from build123d import *

# Parameters (mm, degrees)
SKETCH1_R           = 12
BOSS_EXTRUDE1_DEPTH = 20
CUT_EXTRUDE1_DEPTH  = 13
SKETCH3_R           = 3
CUT_EXTRUDE2_DEPTH  = 13


with BuildPart() as part:
    # Sketch1 → Boss-Extrude1 (new body)
    with BuildSketch(Plane(origin=(0, 0, 0), x_dir=(1, 0, 0), z_dir=(0, 1, 0))):
        with Locations(Location((0, 0, 0), (0, 0, 270))):
            Circle(SKETCH1_R)
    extrude(amount=BOSS_EXTRUDE1_DEPTH)

    # Sketch2 → Cut-Extrude1 (cut)
    with BuildSketch(Plane.XZ):
        with BuildLine():
            Line((3.05, 2.739981752), (3.05, -2.739981752))
            ThreePointArc((3.05, -2.739981752), (-4.1, 0), (3.05, 2.739981752))
        make_face()
    extrude(amount=-CUT_EXTRUDE1_DEPTH, mode=Mode.SUBTRACT)

    # Sketch3 → Cut-Extrude2 (cut)
    with BuildSketch(Plane(origin=(0, 20, 0), x_dir=(1, 0, 0), z_dir=(0, 1, 0))):
        with Locations(Location((0, 0, 0), (0, 0, 270))):
            Circle(SKETCH3_R)
    extrude(amount=-CUT_EXTRUDE2_DEPTH, mode=Mode.SUBTRACT)


solid = part.part
Design review of the part built by this model. Coordinates are the model's own, in mm. A direction names the side the tool comes from. Round coordinates to 2 decimals unless told otherwise and drop trailing zeros. Loops run counter-clockwise (first coordinate to the right, second up) from the corner with the lowest first, then second, coordinate; pieces in that order, holes last. Notation, with made-up numbers: (71.5, 6.5) - (82.5, 6.5) arc R6 cw to (82.5, 17.5) - close; hole circle Ø5 at (72.25, 75). An arc over 180 degrees is marked (long way). One line per item, written item: value. Start each with the question number.
1) Consider section C-C on y = 18.25. Give the boundary of the cut face in (x, z), then the cut area to 3 significant figures.
2) Insertion check: pin 1 Ø2 at (x, z) = (1, 2) entering from -Y; pin 2 Ø3 at (x, y) = (6.5, 4.5) entering from +Z; pin 3 Ø1 at (y, z) = (13, -8) entering from +X. Each pin has a flat end and moves straight along its axis. Give the tip position at first contact, or say it passes through.
3) Draft analysis for pull direction Z (two halves, no side actions). For faces 3 (the cylindrical face through (3.604, 9.86, 11.446)), 4 (the flat face through (0, 0, 5)), 5 (the cylindrical face through (0.9, 16.55, 2.86)), state which applies: +Z half, -Z half, draft (parallel to the pull), parting line (faces both ways), or undercut.
4) To check wall thickness, follow L1, parallel to X at y = 15.5, z = 0; L2, parallel to X at y = 4.5, z = 0; L3, parallel to Z at x = 2.75, y = 18. State the ranges of each line that lie inside material, in increasing order. Write a range as from..to.
5) Consider section D-D on x = 9.25. Give the boundary of the cut face in (y, z), then the cut area to 3 significant figures.
6) Consider section A-A on x = 0. Give the boundary of the cut face in (y, z).
7) Consider section B-B on z = 0. Give the boundary of the cut face in (x, y).
8) For faces 1 (the flat face through (-2.5, 20, 2.5)), 2 (the flat face through (-3, 13, 1)), list the 3-axis set-ups (+Z, -Z, +X, -X, +Y, -Y) from which the entire face can be reached by the end or side of a thin tool; tool diameter is ignored.
Reported:
1. outline: circle Ø24 at (0, 0); hole circle Ø6 at (0, 0)
1. area: 424 mm^2
2. pin 1: stops at y = 13
2. pin 2: stops at z = 10.91
2. pin 3: stops at x = 9.37
3. face 3: parting line
3. face 4: draft
3. face 5: undercut
4. L1: x = -12..-3, 3..12
4. L2: x = -12..-4.1, 3.05..12
4. L3: z = -11.68..-1.2, 1.2..11.68
5. outline: (0, -7.64) - (20, -7.64) - (20, 7.64) - (0, 7.64) - close
5. area: 306 mm^2
6. outline: (0, -12) - (20, -12) - (20, -3) - (13, -3) - (13, -4.1) - (0, -4.1) - close; (0, 4.1) - (13, 4.1) - (13, 3) - (20, 3) - (20, 12) - (0, 12) - close
7. outline: (-12, 0) - (-4.1, 0) - (-4.1, 13) - (-3, 13) - (-3, 20) - (-12, 20) - close; (3, 13) - (3.05, 13) - (3.05, 0) - (12, 0) - (12, 20) - (3, 20) - close
8. face 1: +Z, -Z, +X, -X, +Y
8. face 2: -Y
